from build123d import *

# Parameters (mm, degrees)
BOSS_EXTRUDE1_DEPTH = 1
BOSS_EXTRUDE2_DEPTH = 3


with BuildPart() as part:
    # Sketch2 → Boss-Extrude1 (new body)
    with BuildSketch(Plane(origin=(0, 0, 0), x_dir=(1, 0, 0), z_dir=(0, 1, 0))):
        Polygon((17.320508076, 0), (8.660254038, 15), (-8.660254038, 15), (-17.320508076, 0), (-8.660254038, -15), (8.660254038, -15), align=None)
        Polygon((8.660254038, 0), (4.330127019, 7.5), (-4.330127019, 7.5), (-8.660254038, 0), (-4.330127019, -7.5), (4.330127019, -7.5), align=None, mode=Mode.SUBTRACT)
    extrude(amount=BOSS_EXTRUDE1_DEPTH)

    # Sketch2_2 → Boss-Extrude2 (add)
    with BuildSketch(Plane(origin=(0, 0, 0), x_dir=(1, 0, 0), z_dir=(0, 1, 0))):
        Polygon((-4.330127019, -7.5), (4.330127019, -7.5), (8.660254038, 0), (4.330127019, 7.5), (-4.330127019, 7.5), (-8.660254038, 0), align=None)
    extrude(amount=BOSS_EXTRUDE2_DEPTH)


solid = part.part
For this review, take the finished solid that the model builds, in its own axes (mm). A direction names the side the tool comes from. Round coordinates to 2 decimals unless told otherwise and drop trailing zeros. Write each loop counter-clockwise with the first axis right and the second up, starting at its lowest first coordinate (ties: lowest second). Pieces come first, ordered by that corner, then holes. Notation, with made-up numbers: (10, 18) - (14, 18) arc R18 ccw to (14, 42) - close; hole circle Ø4 at (14.5, 23). An arc over 180 degrees is marked (long way). Write item = value, one per line. Start each with the question number.
1. Consider section C-C on z = -0.75. State the section outline as (x, y) points, plus the area to 3 significant figures.
2. Consider section A-A on x = 2.5. State the section outline as (y, z) points.
3. Consider section D-D on y = 2.3. State the section outline as (x, z) points, plus the area to 3 significant figures.
4. Consider section B-B on y = 0.6. State the section outline as (x, z) points.
5. For pin 1 Ø1.5 at (y, z) = (0.5, 3.5) entering from +X, flat-tipped, find the tip position at first contact; note if it passes through.
6. For faces 1 (the face through (0, 2, -7.5)), 2 (the face through (-6.526, 1.986, 3.698)), 3 (the face through (7, 1, -4)), 4 (the face through (0, 2, 7.5)), list the 3-axis set-ups (+Z, -Z, +X, -X, +Y, -Y) from which the entire face can be reached by the end or side of a thin tool; tool diameter is ignored.
7. Wall thickness on L1, parallel to Z at x = 0.5, y = 1.5; L2, parallel to Y at x = -9.5, z = 11.25; L3, parallel to Z at x = -5, y = 1.35: over which ranges is each line inside the solid? List them lowest first.
Evaluation:
q1.outline = (-16.89, 0) - (16.89, 0) - (16.89, 1) - (8.23, 1) - (8.23, 3) - (-8.23, 3) - (-8.23, 1) - (-16.89, 1) - close
q1.area = 66.7 mm2
q2.outline = (0, -15) - (1, -15) - (1, -7.5) - (3, -7.5) - (3, 7.5) - (1, 7.5) - (1, 15) - (0, 15) - close
q3.outline = (-8.66, 0) - (-4.33, -7.5) - (4.33, -7.5) - (8.66, 0) - (4.33, 7.5) - (-4.33, 7.5) - close
q3.area = 195 mm2
q4.outline = (-17.32, 0) - (-8.66, -15) - (8.66, -15) - (17.32, 0) - (8.66, 15) - (-8.66, 15) - close
q5.pin_1 = 15.73
q6.face_1 = -Z, +X, -X, +Y
q6.face_2 = +Z, -X, +Y
q6.face_3 = +Y
q6.face_4 = +Z, +X, -X, +Y
q7.L1 = -7.5 to 7.5
q7.L2 = 0 to 1
q7.L3 = -6.34 to 6.34
